from build123d import *

# Parameters (mm, degrees)
PAD002_DEPTH         = 350
POCKET001_DEPTH      = 8.001
POCKET001_DEPTH_BACK = 30.001
SKETCH_W             = 12
SKETCH_H             = 12
POCKET_DEPTH         = 264.001
POCKET_DEPTH_BACK    = 264.001


with BuildPart() as part:
    # Sketch003 → Pad002 (new body, symmetric)
    with BuildSketch(Plane.XZ):
        Polygon((214.5, 0), (218.5, 0), (218.5, -8), (226.5, -8), (226.5, 25.632357), (214.5, 30), align=None)
    extrude(amount=PAD002_DEPTH, both=True)

    # Sketch004 → Pocket001 (cut, two sides)
    with BuildSketch(Plane.XY) as pocket001_sk:
        Polygon((226.5, -350), (226.5, -264), (214.5, -252), (214.5, -350), align=None)
        Polygon((226.5, 350), (226.5, 264), (214.5, 252), (214.5, 350), align=None)
    extrude(amount=-POCKET001_DEPTH, mode=Mode.SUBTRACT)
    extrude(pocket001_sk.sketch, amount=POCKET001_DEPTH_BACK, mode=Mode.SUBTRACT)

    # Sketch → Pocket (cut, two sides)
    with BuildSketch(Plane.XZ) as pocket_sk:
        with Locations((220.5, 24)):
            Rectangle(SKETCH_W, SKETCH_H)
    extrude(amount=-POCKET_DEPTH, mode=Mode.SUBTRACT)
    extrude(pocket_sk.sketch, amount=POCKET_DEPTH_BACK, mode=Mode.SUBTRACT)


solid = part.part
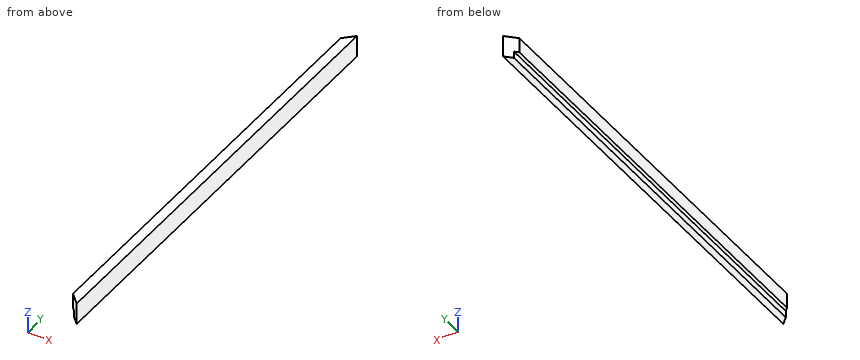
Geometry check sheet. Reference: the model listing, model coordinates, mm. Round coordinates to 2 decimals unless told otherwise and drop trailing zeros. Write each loop counter-clockwise with the first axis right and the second up, starting at its lowest first coordinate (ties: lowest second). Pieces come first, ordered by that corner, then holes.
Item 1: Go/stop test with flat-tipped pins: pin 1 Ø1 at (x, z) = (219, 4) entering from -Y; pin 2 Ø1.2 at (x, y) = (217, -108) entering from -Z; pin 3 Ø2.5 at (y, z) = (6.5, -2) entering from -X. Record where each tip stops, or that it passes through.
Determined:
pin 1: stops at y = -257
pin 2: stops at z = 0
pin 3: stops at x = 218.5
Item 2: Section check B-B (z = 6.5). Record the boundary of the cut face in (x, y).
Determined:
outline: (214.5, -252) - (226.5, -264) - (226.5, 264) - (214.5, 252) - close
Item 3: Section check C-C (x = 216.5). Record the boundary of the cut face in (y, z).
Determined:
outline: (-254, 0) - (254, 0) - (254, 18) - (-254, 18) - close
Item 4: Section check A-A (y = -2). Record the boundary of the cut face in (x, z).
Determined:
outline: (214.5, 0) - (218.5, 0) - (218.5, -8) - (226.5, -8) - (226.5, 18) - (214.5, 18) - close
Item 5: Material ranges on line 1 along X through (y, z) = (-15, -0.5); line 2 along Z through (x, y) = (218, -211.5); line 3 along Y through (x, z) = (219.5, 14), recorded low to high.
Determined:
line 1: x = 218.5 to 226.5
line 2: z = 0 to 18
line 3: y = -257 to 257
